Design review of the part built by this model. Coordinates are the model's own, in mm. A direction names the side the tool comes from. Coordinates: 2 decimals unless noted, no trailing zeros. Order: outer loops, then holes, each group sorted by start corner. A loop starts at its lowest first (then second) coordinate and runs counter-clockwise, first axis right, second up. Notation, with made-up numbers: (13, 41) -> (66, 41) arc R18 cw to (66, 65) -> close; hole circle Ø3 at (-38.5, -19). An arc over 180 degrees is marked (long way). Write item = value, one per line.
```python
from build123d import *

# Parameters (mm, degrees)
CROQUIS1_W              = 1300
CROQUIS1_H              = 25.535714286
SALIENTE_EXTRUIR1_DEPTH = 500
CROQUIS2_R              = 25.810333558
CROQUIS2_R_2            = 25.368411914
CROQUIS2_R_3            = 27.841445981
CROQUIS2_R_4            = 26.795222898
CROQUIS2_R_5            = 27.244240978
SALIENTE_EXTRUIR2_DEPTH = 500


with BuildPart() as part:
    # Croquis1 → Saliente-Extruir1 (new body)
    with BuildSketch(Plane.XY):
        with Locations((-33.200611326, 136.964285714)):
            Rectangle(CROQUIS1_W, CROQUIS1_H)
    extrude(amount=SALIENTE_EXTRUIR1_DEPTH)

    # Croquis2 → Saliente-Extruir2 (add)
    with BuildSketch(Plane.XZ.offset(-124.196428571)):
        with Locations((-606.046625582, 435.691010879)):
            Circle(CROQUIS2_R)
        with Locations((-606.046625582, 61.441174281)):
            Circle(CROQUIS2_R_2)
        with Locations((-13.842861157, 435.691010879)):
            Circle(CROQUIS2_R)
        with Locations((522.438513892, 435.691010879)):
            Circle(CROQUIS2_R_3)
        with Locations((-13.842861157, 61.441174281)):
            Circle(CROQUIS2_R_4)
        with Locations((522.438513892, 61.441174281)):
            Circle(CROQUIS2_R_5)
    extrude(amount=SALIENTE_EXTRUIR2_DEPTH)


solid = part.part
```
(1) We need section C-C (z = 189.5). Write out the cut boundary in (x, y).
Report:
outline = (-683.2, 124.2) -> (616.8, 124.2) -> (616.8, 149.73) -> (-683.2, 149.73) -> close
(2) Insertion check: pin 1 (4 mm diameter, centred on x = 151, z = 415.5, fed in from -Y); pin 2 (2 mm diameter, centred on y = -308.5, z = 63, fed in from +X). Each pin has a flat end and moves straight along its axis. Give the tip position at first contact, or say it passes through.
Report:
pin_1 = 124.2
pin_2 = 549.68
(3) For L1, parallel to Z at x = -608, y = -192.5; L2, parallel to X at y = -202.5, z = 56.5; L3, parallel to X at y = -269, z = 431, list the stretches that pass through material, from the lowest coordinate up.
Report:
L1 = 36.15 to 86.73, 409.95 to 461.43
L2 = -630.93 to -581.16, -40.18 to 12.49, 495.65 to 549.23
L3 = -631.43 to -580.67, -39.22 to 11.54, 495 to 549.88
(4) The part is to be moulded in two halves that separate along Z. For faces 3 (the flat face through (-42, 137, 0)), 4 (the cylindrical face through (-17.203, -122.304, 461.282)), 5 (the flat face through (-683.201, 137, 246)), say which applies: released by +Z, released by -Z, zero draft, split by the parting line, or undercut.
Report:
face_3 = released by -Z
face_4 = undercut
face_5 = zero draft
(5) We need section A-A (x = -509.5). Write out the cut boundary in (y, z).
Report:
outline = (124.2, 0) -> (149.73, 0) -> (149.73, 500) -> (124.2, 500) -> close
(6) For faces 1 (the cylindrical face through (-582.613, -122.304, 51.725)), 2 (the flat face through (-606, -375.804, 436)), list the 3-axis set-ups (+Z, -Z, +X, -X, +Y, -Y) from which the entire face can be reached by the end or side of a thin tool; tool diameter is ignored.
Report:
face_1 = -Y
face_2 = +Z, -Z, +X, -X, -Y
(7) We need section B-B (y = -230). Write out the cut boundary in (x, z), and give its area (3 significant figures).
Report:
outline = circle Ø51.62 at (-606.05, 435.69); circle Ø50.74 at (-606.05, 61.44); circle Ø53.59 at (-13.84, 61.44); circle Ø51.62 at (-13.84, 435.69); circle Ø55.68 at (522.44, 435.69); circle Ø54.49 at (522.44, 61.44)
area = 13,200 mm²
